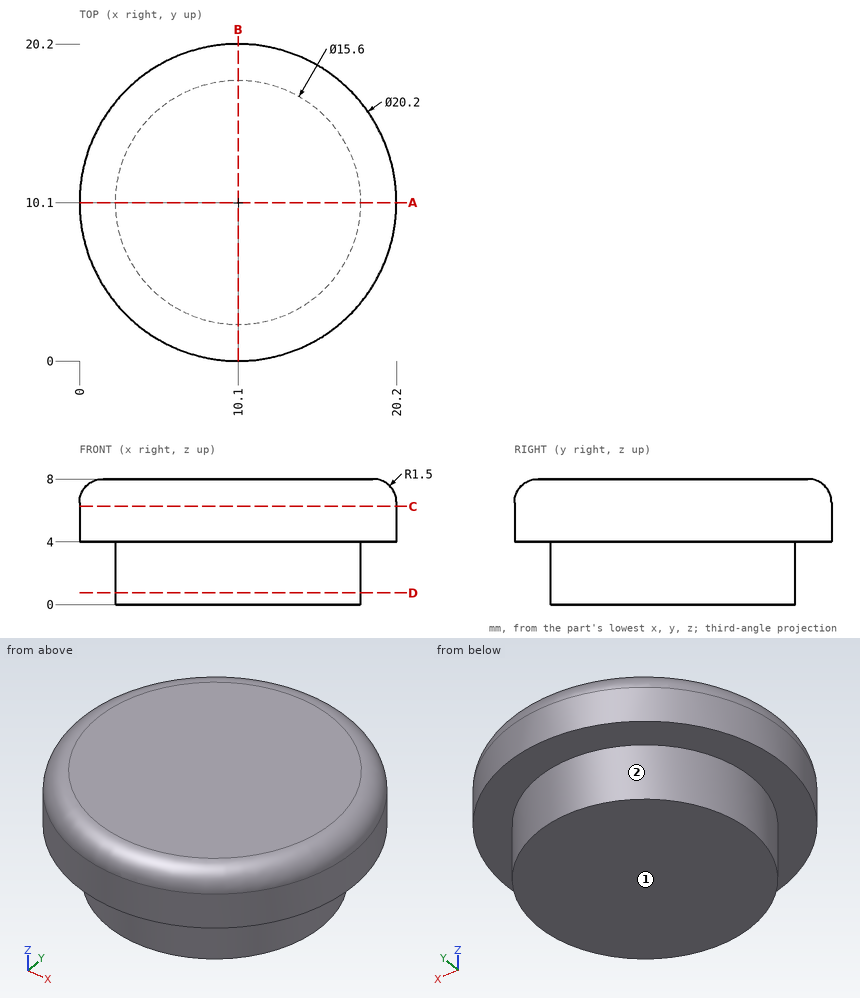
For this review, use the dimensioned drawing (mm, ordinates from the lowest corner) and the shaded views. A direction names the side the tool comes from. Round coordinates to 2 decimals unless told otherwise and drop trailing zeros. Write each loop counter-clockwise with the first axis right and the second up, starting at its lowest first coordinate (ties: lowest second). Pieces come first, ordered by that corner, then holes. Notation, with made-up numbers: M -12,-1 L 42,-1 A18 ccw 42,17 Z; hole C 15,23.25 d5. An arc over 180 degrees is marked long. Write item = value, one per line. Start each with the question number.
(1) We need section A-A (y = 10.1). Give the boundary of the cut face in (x, z).
(2) For the marked faces 1 and 2, list the 3-axis set-ups (+Z, -Z, +X, -X, +Y, -Y) from which the entire face can be reached by the end or side of a thin tool; tool diameter is ignored.
(3) We need section C-C (z = 6.25). Give the boundary of the cut face in (x, y), then the cut area to 3 significant figures.
(4) We need section D-D (z = 0.75). Give the boundary of the cut face in (x, y), then the cut area to 3 significant figures.
(5) For line 1 along Z through (x, y) = (2.5, 13.5); line 2 along Y through (x, z) = (8.5, 6.25); line 3 along Y through (x, z) = (11.5, 1.5), list the stretches that pass through material, from the lowest coordinate up.
(6) Clearance check with flat-ended pins moving along their axes: pin 1 Ø1.5 at (y, z) = (15.5, 7) entering from +X; pin 2 Ø3 at (x, z) = (18, 7) entering from +Y; pin 3 Ø2 at (x, z) = (18, 2.5) entering from -Y. State where each tip first meets the part, or that it passes through.
Results found:
q1.outline = M 0,4 L 2.3,4 L 2.3,0 L 17.9,0 L 17.9,4 L 20.2,4 L 20.2,6.5 A1.5 ccw 18.7,8 L 1.5,8 A1.5 ccw 0,6.5 Z
q2.face_1 = -Z, +X, -X, +Y, -Y
q2.face_2 = -Z
q3.outline = C 10.1,10.1 d20.2
q3.area = 320 mm²
q4.outline = C 10.1,10.1 d15.6
q4.area = 191 mm²
q5.line_1 = 4 to 8
q5.line_2 = 0.13 to 20.07
q5.line_3 = 2.43 to 17.77
q6.pin_1 = 19.02
q6.pin_2 = 17.87
q6.pin_3 = 6.46
